For this review, take the finished solid that the model builds, in its own axes (mm). Face numbers are marked on the shaded views. A direction names the side the tool comes from. Coordinates: 2 decimals unless noted, no trailing zeros. Order: outer loops, then holes, each group sorted by start corner. A loop starts at its lowest first (then second) coordinate and runs counter-clockwise, first axis right, second up. Notation, with made-up numbers: (37, 82) -> (71, 82) arc R14 ccw to (71, 94) -> close; hole circle Ø9 at (81, -33). An arc over 180 degrees is marked (long way). Write item = value, one per line. Start each with the question number.
1) Insertion check: pin 1 Ø4.5 at (y, z) = (7, 39) entering from +X; pin 2 Ø14 at (x, y) = (42.5, 2) entering from -Z; pin 3 Ø5.5 at (x, y) = (36.5, 1) entering from +Z; pin 4 Ø2.5 at (y, z) = (5, -36) entering from -X. Each pin has a flat end and moves straight along its axis. Give the tip position at first contact, or say it passes through.
2) Wall thickness on probe 1 along Z at (x, y) = (1.35, 5); probe 2 along Y at (x, z) = (1.35, -36); probe 3 along Z at (x, y) = (2.95, 5): over which ranges is each line inside the solid? List them lowest first. Write a range as [from, to].
3) Machinability: for the marked faces 4, 5 and 6, which of the approach directions +Z, -Z, +X, -X, +Y, -Y give a long, thin tool a straight path to every point of the face, cutting with its end or side? Answer none if there is none.
4) Consider section B-B on x = 16.5. Give the boundary of the cut face in (y, z), and give its area (3 significant figures).
5) Draft analysis for pull direction Z (two halves, no side actions). For the marked faces 1, 2 and 3, state which applies: +Z half, -Z half, draft (parallel to the pull), parting line (faces both ways), or undercut.
6) Consider section A-A on z = 1.5. Give the boundary of the cut face in (x, y), and give its area (3 significant figures).
7) Consider section D-D on z = 22.5. Give the boundary of the cut face in (x, y).
8) Consider section C-C on z = 36.5. Give the boundary of the cut face in (x, y), and give its area (3 significant figures).
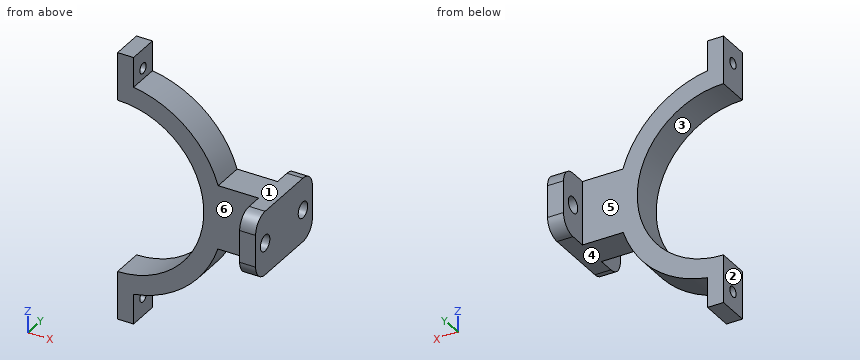
Autodesk Inventor part; units mm, degrees
ref_plane "YZ Plane" through (0, 0, 0) normal (1, 0, 0) x (0, 1, 0)
ref_plane "XZ Plane" through (0, 0, 0) normal (0, 1, 0) x (-1, 0, 0)
ref_plane "XY Plane" through (0, 0, 0) normal (0, 0, 1) x (1, 0, 0)
sketch "Sketch1" plane through (0, 0, 0) normal (0, 1, 0) x (-1, 0, 0)
  arc A0 (0, 27) -> (0, -27) centre (0, 0) ccw
  line L0 (-49.15, 9.8171) -> (-49.15, -10.1829)
  line L1 (-49.15, -10.1829) -> (-31.3896, -10.1829)
  line L2 (-31.5059, 9.8171) -> (-49.15, 9.8171)
  arc A1 (0, 33) -> (-31.5059, 9.8171) centre (0, 0) ccw
  arc A2 (-31.3896, -10.1829) -> (0, -33) centre (0, 0) ccw
  line L3 (0, -33) -> (0, -27)
  line L4 (0, 27) -> (0, 33)
  point P0 (-41.2646, -10.1829)
  point P1 (-41.2646, 9.8171)
  point P2 (27.2866, 9.8171)
  point P3 (26.6483, -10.1829)
  dimension "d0" = 54
  dimension "d33" = 49.15
  dimension "d36" = 20
  dimension "d41" = 33
  dimension "d42" = 33
extrude "Extrusion1" add sketch "Sketch1" along normal blind 10
sketch "Sketch4" plane through (0, 10, 0) normal (0, 1, 0) x (1, 0, 0)
  line L0 (44.15, -9.8171) -> (49.15, -9.8171)
  line L1 (49.15, -9.8171) -> (49.15, 10.1829)
  line L2 (49.15, 10.1829) -> (44.15, 10.1829)
  line L3 (44.15, 10.1829) -> (44.15, -9.8171)
  line L4 (49.15, -9.8171) -> (49.15, 10.1829)
  line L5 (49.15, 10.1829) -> (31.3896, 10.1829)
  line L6 (31.5059, -9.8171) -> (49.15, -9.8171)
  point P0 (0, 0)
  dimension "d16" = 5
extrude "Extrusion3" add sketch "Sketch4" along normal blind 10 and the other way blind 20
sketch "Sketch5" plane through (44.15, 10, -10.1829) normal (-1, 0, 0) x (0, 0, 1)
  circle A0 centre (10, -15) radius 2.5
  circle A1 centre (10, 5) radius 2.5
  line L0 (20, -20) -> (0, -20)
  line L1 (0, 10) -> (20, 10)
  line L2 (0, 0) -> (0, 10)
  line L3 (0, -20) -> (0, -10)
  point P0 (10.1829, -10)
  dimension "d21" = 5
  dimension "d22" = 5
  dimension "d23" = 5
  dimension "d24" = 5
  dimension "d25" = 10
  dimension "d26" = 10
extrude "Extrusion4" cut sketch "Sketch5" against normal blind 10
fillet "Fillet2" radius 5 4 edges at (46.65, -10, 9.8171) (46.65, -10, -10.1829) (46.65, 20, 9.8171) (46.65, 20, -10.1829)
sketch "Sketch7" plane through (0, 0, -33) normal (-1, 0, 0) x (0, 0, 1)
  line L0 (6, 0) -> (6, 10)
  line L1 (6, 10) -> (-9, 10)
  line L2 (-9, 10) -> (-9, 0)
  line L3 (-9, 0) -> (6, 0)
  line L4 (6, 0) -> (6, 10)
  line L5 (6, 10) -> (60, 10)
  line L6 (60, 10) -> (75, 10)
  line L7 (75, 10) -> (75, 0)
  line L8 (75, 0) -> (60, 0)
  line L9 (60, 0) -> (60, 10)
  point P0 (33, 0)
  dimension "d43" = 15
extrude "Extrusion6" add sketch "Sketch7" against normal blind 5
sketch "Sketch8" plane through (5, 0, -33) normal (1, 0, 0) x (0, 0, 1)
  circle A0 centre (-3, -5) radius 1.65
  circle A1 centre (69, -5) radius 1.65
  line L0 (-9, 0) -> (-9, -10)
  line L1 (75, -10) -> (75, 0)
  line L2 (65.619, -10) -> (75, -10)
  line L3 (-9, -10) -> (0.381, -10)
  point P0 (33, 0)
  point P1 (-9, 10)
  point P2 (75, 10)
  point P3 (60, 10)
  point P4 (6, 10)
  dimension "d46" = 6
  dimension "d47" = 6
  dimension "d50" = 3.3
  dimension "d53" = 5
  dimension "d54" = 5
extrude "Extrusion7" cut sketch "Sketch8" against normal blind 5
equation "\"BendRadius\" = Thickness"
equation "\"BendReliefWidth\" = Thickness"
equation "\"BendReliefDepth\" = 0.5 * Thickness"
equation "\"CornerReliefSize\" = 4 * Thickness"
equation "\"MinimumRemnant\" = 2 * Thickness"
equation "\"TransitionRadius\" = BendRadius"
equation "\"JacobiRadiusSize\" = BendRadius"
equation "\"GapSize\" = Thickness"
properties part number "22010_Tube End Support_V1" material "ABS Plastic"
Answer sheet:
q1.pin_1 = 5
q1.pin_2 = -10.18
q1.pin_3 = 9.82
q1.pin_4 = through
q2.probe_1 = [-42, -37.65], [-34.35, -26.97], [26.97, 34.35], [37.65, 42]
q2.probe_2 = [0, 3.35], [6.65, 10]
q2.probe_3 = [-42, -37.65], [-34.35, -26.84], [26.84, 34.35], [37.65, 42]
q3.face_4 = -Z, +X, +Y, -Y
q3.face_5 = +Z, -Z, -X, +Y
q3.face_6 = +Z, -Z, -X, -Y
q4.outline = (0, -28.58) -> (10, -28.58) -> (10, -21.37) -> (0, -21.37) -> close; (0, 21.37) -> (10, 21.37) -> (10, 28.58) -> (0, 28.58) -> close
q4.area = 144 mm2
q5.face_1 = +Z half
q5.face_2 = draft
q5.face_3 = undercut
q6.outline = (26.96, 0) -> (44.15, 0) -> (44.15, -3.15) -> (49.15, -3.15) -> (49.15, 13.15) -> (44.15, 13.15) -> (44.15, 10) -> (26.96, 10) -> close; (44.15, -10) -> (49.15, -10) -> (49.15, -6.85) -> (44.15, -6.85) -> close; (44.15, 16.85) -> (49.15, 16.85) -> (49.15, 20) -> (44.15, 20) -> close
q6.area = 285 mm2
q7.outline = (14.92, 0) -> (24.14, 0) -> (24.14, 10) -> (14.92, 10) -> close
q8.outline = (0, 0) -> (5, 0) -> (5, 3.43) -> (0, 3.43) -> close; (0, 6.57) -> (5, 6.57) -> (5, 10) -> (0, 10) -> close
q8.area = 34.3 mm2
